Work out the finished part from the listing and answer in its coordinate system (mm). Round coordinates to 2 decimals unless told otherwise and drop trailing zeros. Loops run counter-clockwise (first coordinate to the right, second up) from the corner with the lowest first, then second, coordinate; pieces in that order, holes last.
from build123d import *

# Parameters (mm, degrees)
SKETCH1_R           = 4
BOSS_EXTRUDE1_DEPTH = 30
SKETCH2_R           = 2.5
CUT_EXTRUDE1_DEPTH  = 5


with BuildPart() as part:
    # Sketch1 → Boss-Extrude1 (new body)
    with BuildSketch(Plane(origin=(0, 0, 0), x_dir=(0, 0, -1), z_dir=(1, 0, 0))):
        with BuildLine():
            Line((-6, 8), (6, 8))
            Line((6, 8), (6, -8))
            ThreePointArc((6, -8), (0, -14), (-6, -8))
            Line((-6, -8), (-6, 8))
        make_face()
        with Locations((0, -8)):
            Circle(SKETCH1_R, mode=Mode.SUBTRACT)
    extrude(amount=BOSS_EXTRUDE1_DEPTH)

    # Sketch2 → Cut-Extrude1 (cut)
    with BuildSketch(Plane(origin=(0, 8, 0), x_dir=(1, 0, 0), z_dir=(0, 1, 0))):
        with Locations(Location((15, 0, 0), (0, 0, 270))):
            Circle(SKETCH2_R)
    extrude(amount=-CUT_EXTRUDE1_DEPTH, mode=Mode.SUBTRACT)


solid = part.part
Item 1: Section D-D, the plane y = 5.5 is taken. Give the vertices of the cut face in (x, z).
Item 2: Section C-C, the plane y = -11 is taken. Give the vertices of the cut face in (x, z).
Item 3: Determine the mould class of faces 1 (the face through (15, 0, 6)), 2 (the face through (12.56, 5.54, -0.54)), 3 (the face through (15, 3, 0)), 4 (the face through (30, 0, 0)) for opening direction X: pulls with the +X half, pulls with the -X half, needs draft (parallel to the pull), parting line crosses it, or undercut.
Item 4: Each of these flat-tipped pins is pushed along its axis until it touches: P1, Ø1, axis at x = 26.5, z = 4, coming from the -Y side; P2, Ø7, axis at y = -8, z = 0, coming from the +X side (1 decimal). Where does it stop, or does it pass through?
Item 5: Section A-A, the plane x = 15 is taken. Give the vertices of the cut face in (y, z).
Item 6: Straight lines are drawn through the part: line 1 (X direction, y = 4.25, z = 0); line 2 (Y direction, x = 14.25, z = 0); line 3 (Z direction, x = 26.5, y = -8.25). For each, find the intervals that lie inside material, in ascending order.
Item 7: Section B-B, the plane z = 0 is taken. Give the vertices of the cut face in (x, y).
Answer below:
1. outline: (0, -6) - (30, -6) - (30, 6) - (0, 6) - close; hole circle Ø5 at (15, 0)
2. outline: (0, -5.2) - (30, -5.2) - (30, -2.65) - (0, -2.65) - close; (0, 2.65) - (30, 2.65) - (30, 5.2) - (0, 5.2) - close
3. face 1: needs draft
3. face 2: undercut
3. face 3: undercut
3. face 4: pulls with the +X half
4. P1: stops at y = -12.87
4. P2: passes through
5. outline: (-8, -6) - (8, -6) - (8, -2.5) - (3, -2.5) - (3, 2.5) - (8, 2.5) - (8, 6) - (-8, 6) arc R6 ccw to start; hole circle Ø8 at (-8, 0)
6. line 1: x = 0 to 12.5, 17.5 to 30
6. line 2: y = -14 to -12, -4 to 3
6. line 3: z = -5.99 to -3.99, 3.99 to 5.99
7. outline: (0, -14) - (30, -14) - (30, -12) - (0, -12) - close; (0, -4) - (30, -4) - (30, 8) - (17.5, 8) - (17.5, 3) - (12.5, 3) - (12.5, 8) - (0, 8) - close
